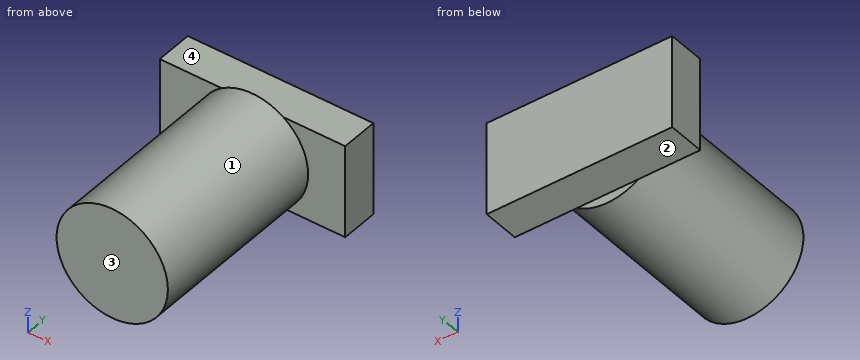
Solid Edge part; units mm, degrees
sketch "Sketch1" plane through (0, 0, 0) normal (0, -1, 0) x (1, 0, 0)
  circle A0 centre (0, 0) radius 3
extrude "Protrusion1" add sketch "Sketch1" against normal blind 10
sketch "Sketch2" plane through (0, 10, 0) normal (0, 1, 0) x (1, 0, 0)
  line L0 (-5, -2.5) -> (5, -2.5)
  line L1 (5, -2.5) -> (5, 2.5)
  line L2 (5, 2.5) -> (-5, 2.5)
  line L3 (-5, 2.5) -> (-5, -2.5)
extrude "ExtrudedProtrusion_3" add sketch "Sketch2" along normal blind 2
Geometry check sheet. Reference: the model listing, model coordinates, mm. Face numbers are marked on the shaded views. A direction names the side the tool comes from. Give positions to 0.01 mm unless a question says otherwise; leave off trailing zeros. Order: outer loops, then holes, each group sorted by start corner. A loop starts at its lowest first (then second) coordinate and runs counter-clockwise, first axis right, second up. Notation, with made-up numbers: (70.25, 20) - (115.25, 20) arc R23 cw to (115.25, 38) - close; hole circle Ø10 at (-26, -9). An arc over 180 degrees is marked (long way). Answer in a Markdown table with one row per item. Add a question column.
Q1. Cross-section at B-B, the plane x = 0. Enter the section's corners in (y, z).
Q2. Cross-section at A-A, the plane z = 0. Enter the section's corners in (x, y), then the cut area to 3 significant figures.
Q3. Gauge pin test, flat ends, axial feed: pin 1 (1 mm diameter, centred on x = 1, y = 11, fed in from -Z); pin 2 (5 mm diameter, centred on x = -2, y = 2, fed in from +Z); pin 3 (3 mm diameter, centred on y = 2.5, z = -1.5, fed in from +X); pin 4 (1 mm diameter, centred on x = 3.5, z = -1, fed in from -Y). Record the tip position at first contact, or that the pin passes through.
Q4. Tool access check on the marked faces 1, 2, 3 and 4. Record the directions out of +Z, -Z, +X, -X, +Y, -Y that give a thin tool (end or side, any length) a straight path to the whole face; none if there is none.
Q5. Cross-section at D-D, the plane x = 4.25. Enter the section's corners in (y, z).
Q6. Cross-section at C-C, the plane y = 3.5. Enter the section's corners in (x, z).
Q7. Material ranges on probe 1 along Y at (x, z) = (-3.5, 1.8); probe 2 along Z at (x, y) = (0.5, 1); probe 3 along X at (y, z) = (1, 2.05), recorded low to high. Write a range as from..to.
Check values:
| question | item | result |
|---|---|---|
| 1 | outline | (0, -3) - (10, -3) - (10, -2.5) - (12, -2.5) - (12, 2.5) - (10, 2.5) - (10, 3) - (0, 3) - close |
| 2 | outline | (-5, 10) - (-3, 10) - (-3, 0) - (3, 0) - (3, 10) - (5, 10) - (5, 12) - (-5, 12) - close |
| 2 | area | 80.0 mm^2 |
| 3 | pin 1 | stops at z = -2.5 |
| 3 | pin 2 | stops at z = 3 |
| 3 | pin 3 | stops at x = 3 |
| 3 | pin 4 | stops at y = 10 |
| 4 | face 1 | -Y |
| 4 | face 2 | -Z, +X, -X, +Y |
| 4 | face 3 | +Z, -Z, +X, -X, -Y |
| 4 | face 4 | +Z, +X, -X, +Y |
| 5 | outline | (10, -2.5) - (12, -2.5) - (12, 2.5) - (10, 2.5) - close |
| 6 | outline | circle Ø6 at (0, 0) |
| 7 | probe 1 | y = 10..12 |
| 7 | probe 2 | z = -2.96..2.96 |
| 7 | probe 3 | x = -2.19..2.19 |
